Autodesk Inventor part; units mm, degrees
ref_plane "YZ Plane" through (0, 0, 0) normal (1, 0, 0) x (0, 1, 0)
ref_plane "XZ Plane" through (0, 0, 0) normal (0, 1, 0) x (-1, 0, 0)
ref_plane "XY Plane" through (0, 0, 0) normal (0, 0, 1) x (1, 0, 0)
sketch "スケッチ1" plane through (0, 0, 0) normal (0, 0, 1) x (1, 0, 0)
  line L0 (-12.25, 11.25) -> (12.25, 11.25)
  line L1 (14.25, 9.25) -> (14.25, -33.25)
  line L2 (12.25, -35.25) -> (-12.25, -35.25)
  line L3 (-14.25, -33.25) -> (-14.25, 9.25)
  line L4 (-12.25, 11.25) -> (-14.25, 9.25)
  line L5 (12.25, 11.25) -> (14.25, 9.25)
  line L6 (14.25, -33.25) -> (12.25, -35.25)
  line L7 (-12.25, -35.25) -> (-14.25, -33.25)
  line L8 (0, 0) -> (-26.5626, 0) construction
  line L9 (0, 0) -> (0, 27.9433) construction
  line L10 (-11, 8) -> (11, 8) construction
  line L11 (11, 8) -> (11, -32) construction
  line L12 (11, -32) -> (-11, -32) construction
  line L13 (-11, -32) -> (-11, 8) construction
  line L14 (-13.15, -28.5) -> (-13.15, 4.5)
  line L15 (-7.5, 10.15) -> (7.5, 10.15)
  line L16 (13.15, 4.5) -> (13.15, -28.5)
  line L17 (7.5, -34.15) -> (-7.5, -34.15)
  line L18 (8.5, 8) -> (8.5, 9.15)
  line L19 (11, 5.5) -> (12.15, 5.5)
  arc A0 (8.5, 8) -> (11, 5.5) centre (11, 8) ccw
  line L20 (12.15, -29.5) -> (11, -29.5)
  line L21 (8.5, -32) -> (8.5, -33.15)
  arc A1 (11, -29.5) -> (8.5, -32) centre (11, -32) ccw
  line L22 (-8.5, 8) -> (-8.5, 9.15)
  line L23 (-11, 5.5) -> (-12.15, 5.5)
  arc A2 (-11, 5.5) -> (-8.5, 8) centre (-11, 8) ccw
  line L24 (-12.15, -29.5) -> (-11, -29.5)
  line L25 (-8.5, -32) -> (-8.5, -33.15)
  arc A3 (-8.5, -32) -> (-11, -29.5) centre (-11, -32) ccw
  arc A4 (8.5, 9.15) -> (7.5, 10.15) centre (7.5, 9.15) ccw
  arc A5 (13.15, 4.5) -> (12.15, 5.5) centre (12.15, 4.5) ccw
  arc A6 (12.15, -29.5) -> (13.15, -28.5) centre (12.15, -28.5) ccw
  arc A7 (7.5, -34.15) -> (8.5, -33.15) centre (7.5, -33.15) ccw
  arc A8 (-8.5, -33.15) -> (-7.5, -34.15) centre (-7.5, -33.15) ccw
  arc A9 (-13.15, -28.5) -> (-12.15, -29.5) centre (-12.15, -28.5) ccw
  arc A10 (-12.15, 5.5) -> (-13.15, 4.5) centre (-12.15, 4.5) ccw
  arc A11 (-7.5, 10.15) -> (-8.5, 9.15) centre (-7.5, 9.15) ccw
  point P0 (-14.25, 11.25)
  point P1 (14.25, -35.25)
  point P2 (14.25, 11.25)
  point P3 (-14.25, -35.25)
  point P4 (8.5, 10.15)
  point P5 (13.15, 5.5)
  point P6 (13.15, -29.5)
  point P7 (8.5, -34.15)
  point P8 (-8.5, 10.15)
  point P9 (-13.15, 5.5)
  point P10 (-13.15, -29.5)
  point P11 (-8.5, -34.15)
  dimension "d0" = 2
  dimension "d1" = 2
  dimension "d2" = 2
  dimension "d3" = 2
  dimension "d4" = 2
  dimension "d5" = 2
  dimension "d6" = 2
  dimension "d7" = 2
  dimension "d8" = 28.5
  dimension "d9" = 11.25
  dimension "d10" = 46.5
  dimension "d11" = 8
  dimension "d12" = 22
  dimension "d13" = 40
  dimension "d14" = 1.1
  dimension "d15" = 2.5
  dimension "d16" = 2.5
  dimension "d17" = 1.1
  dimension "d18" = 1.1
  dimension "d19" = 1
extrude "押し出し1" add sketch "スケッチ1" along normal blind 3.1
hole "穴1" at (-11, 8, 0) at (11, 8, 0) at (11, -32, 0) at (-11, -32, 0) direction (0, 0, 1) diameter 2.5 end through all
sketch "スケッチ3" plane through (0, 0, 0) normal (0, 0, -1) x (-1, 0, 0)
  line L0 (-12.25, 11.25) -> (12.25, 11.25) construction
  line L1 (12.25, 11.25) -> (14.25, 9.25) construction
  line L2 (14.25, 9.25) -> (14.25, -33.25) construction
  line L3 (14.25, -33.25) -> (12.25, -35.25) construction
  line L4 (12.25, -35.25) -> (-12.25, -35.25) construction
  line L5 (-12.25, -35.25) -> (-14.25, -33.25) construction
  line L6 (-14.25, -33.25) -> (-14.25, 9.25) construction
  line L7 (-14.25, 9.25) -> (-12.25, 11.25) construction
  line L8 (11.087, 10.625) -> (-11.087, 10.625)
  line L9 (-11.9911, 10.625) -> (-13.625, 8.9911) construction
  line L10 (-13.625, 8.087) -> (-13.625, -32.087)
  line L11 (-13.625, -32.9911) -> (-11.9911, -34.625) construction
  line L12 (-11.087, -34.625) -> (11.087, -34.625)
  line L13 (11.9911, -34.625) -> (13.625, -32.9911) construction
  line L14 (13.625, -32.087) -> (13.625, 8.087)
  line L15 (13.625, 8.9911) -> (11.9911, 10.625) construction
  line L16 (-13.1857, -33.1476) -> (-12.1476, -34.1857)
  line L17 (12.1476, -34.1857) -> (13.1857, -33.1476)
  line L18 (12.1476, 10.1857) -> (13.1857, 9.1476)
  line L19 (-13.1857, 9.1476) -> (-12.1476, 10.1857)
  arc A0 (-13.1857, 9.1476) -> (-13.625, 8.087) centre (-12.125, 8.087) ccw
  arc A1 (-11.087, 10.625) -> (-12.1476, 10.1857) centre (-11.087, 9.125) ccw
  arc A2 (12.1476, 10.1857) -> (11.087, 10.625) centre (11.087, 9.125) ccw
  arc A3 (13.625, 8.087) -> (13.1857, 9.1476) centre (12.125, 8.087) ccw
  arc A4 (13.1857, -33.1476) -> (13.625, -32.087) centre (12.125, -32.087) ccw
  arc A5 (11.087, -34.625) -> (12.1476, -34.1857) centre (11.087, -33.125) ccw
  arc A6 (-12.1476, -34.1857) -> (-11.087, -34.625) centre (-11.087, -33.125) ccw
  arc A7 (-13.625, -32.087) -> (-13.1857, -33.1476) centre (-12.125, -32.087) ccw
  arc A8 (-12.15, 5.5) -> (-13.15, 4.5) centre (-12.15, 4.5) ccw
  line L20 (-12.15, 5.5) -> (-11, 5.5)
  arc A9 (-11, 5.5) -> (-8.5, 8) centre (-11, 8) ccw
  line L21 (-8.5, 8) -> (-8.5, 9.15)
  arc A10 (-7.5, 10.15) -> (-8.5, 9.15) centre (-7.5, 9.15) ccw
  line L22 (-7.5, 10.15) -> (7.5, 10.15)
  arc A11 (8.5, 9.15) -> (7.5, 10.15) centre (7.5, 9.15) ccw
  line L23 (8.5, 9.15) -> (8.5, 8)
  arc A12 (8.5, 8) -> (11, 5.5) centre (11, 8) ccw
  line L24 (11, 5.5) -> (12.15, 5.5)
  arc A13 (13.15, 4.5) -> (12.15, 5.5) centre (12.15, 4.5) ccw
  circle A14 centre (11, 8) radius 1.25
  line L25 (13.15, 4.5) -> (13.15, -28.5)
  arc A15 (12.15, -29.5) -> (13.15, -28.5) centre (12.15, -28.5) ccw
  line L26 (12.15, -29.5) -> (11, -29.5)
  arc A16 (11, -29.5) -> (8.5, -32) centre (11, -32) ccw
  line L27 (8.5, -32) -> (8.5, -33.15)
  arc A17 (7.5, -34.15) -> (8.5, -33.15) centre (7.5, -33.15) ccw
  circle A18 centre (11, -32) radius 1.25
  line L28 (7.5, -34.15) -> (-7.5, -34.15)
  arc A19 (-8.5, -33.15) -> (-7.5, -34.15) centre (-7.5, -33.15) ccw
  line L29 (-8.5, -33.15) -> (-8.5, -32)
  arc A20 (-8.5, -32) -> (-11, -29.5) centre (-11, -32) ccw
  line L30 (-11, -29.5) -> (-12.15, -29.5)
  arc A21 (-13.15, -28.5) -> (-12.15, -29.5) centre (-12.15, -28.5) ccw
  circle A22 centre (-11, -32) radius 1.25
  line L31 (-13.15, -28.5) -> (-13.15, 4.5)
  circle A23 centre (-11, 8) radius 1.25
  point P0 (0, 0)
  dimension "d30" = 0.625
  dimension "d31" = 1.5
  dimension "d32" = 0.2
extrude "押し出し2" add sketch "スケッチ3" along normal blind 0.75
properties part number "COXA_YAW_ROLL_ADPT_SPACER_2"
Work out the finished part from the listing and answer in its coordinate system (mm). A direction names the side the tool comes from. Coordinates: 2 decimals unless noted, no trailing zeros. Write each loop counter-clockwise with the first axis right and the second up, starting at its lowest first coordinate (ties: lowest second). Pieces come first, ordered by that corner, then holes. Notation, with made-up numbers: M 79.5,10.25 L 120.5,10.25 A22 ccw 120.5,19.25 Z; hole C 42,-25.5 d7. An arc over 180 degrees is marked long. Use one line per item in the form item = value. Start each with the question number.
1. Straight lines are drawn through the part: probe 1 along X at (y, z) = (8, 0.65); probe 2 along Y at (x, z) = (-11, 0.95); probe 3 along X at (y, z) = (8, -0.3) (3 decimals). For each, find the intervals that lie inside material, in ascending order. Write a range as from..to.
2. This flat-tipped pin is pushed along its axis until it touches: P1, Ø0.8, axis at x = 2.5, z = -0.5, coming from the -Y side (3 decimals). Where does it stop, or does it pass through?
3. The mould has two halves that part along Y. Classify faces 1 (the face through (12, 5.5, 1)), 2 (the face through (13.2, 10.3, 1.5)), 3 (the face through (9.9, -31.41, 1.2)), 4 (the face through (-14.25, -12, 2)): released by +Y, released by -Y, zero draft, split by the parting line, or undercut.
4. The part is cut by section C-C (z = 1.5). Give the number of separate pieces and of enclosed holes in the cut face, plus the area to 3 significant figures.
5. The part is cut by section A-A (y = -16.5). Give the vertices of the cut face in (x, z) (3 decimals).
6. A tool of negligible diameter and unlimited length cuts with its end or side. For faces 5 (the face through (12.674, -33.659, -0.37)), 6 (the face through (-12, -29.5, 1)), 7 (the face through (-12.659, -33.674, -0.37)), 8 (the face through (12.674, 9.659, -0.37)), 9 (the face through (-12.659, 9.674, -0.37)), from which of +Z, -Z, +X, -X, +Y, -Y can it reach the whole face along a straight path? Write none if from no direction.
7. The part is cut by section B-B (x = -2.5). Give the vertices of the cut face in (y, z) (3 decimals), plus the area to 3 significant figures.
Evaluation:
q1.probe_1 = -14.25..-12.25, -9.75..-8.5, 8.5..9.75, 12.25..14.25
q1.probe_2 = -35.25..-33.25, -30.75..-29.5, 5.5..6.75, 9.25..11.25
q1.probe_3 = -13.625..-12.25, -9.75..-8.5, 8.5..9.75, 12.25..13.625
q2.P1 = -34.625
q3.face_1 = undercut
q3.face_2 = released by +Y
q3.face_3 = undercut
q3.face_4 = zero draft
q4.separate_pieces = 1
q4.enclosed_holes = 5
q4.area = 215 mm^2
q5.outline = M -14.25,0 L -13.625,0 L -13.625,-0.75 L -13.15,-0.75 L -13.15,3.1 L -14.25,3.1 Z; M 13.15,-0.75 L 13.625,-0.75 L 13.625,0 L 14.25,0 L 14.25,3.1 L 13.15,3.1 Z
q6.face_5 = -Z, +X, -Y
q6.face_6 = +Z, -Z
q6.face_7 = -Z, -X, -Y
q6.face_8 = -Z, +X, +Y
q6.face_9 = -Z, -X, +Y
q7.outline = M -35.25,0 L -34.625,0 L -34.625,-0.75 L -34.15,-0.75 L -34.15,3.1 L -35.25,3.1 Z; M 10.15,-0.75 L 10.625,-0.75 L 10.625,0 L 11.25,0 L 11.25,3.1 L 10.15,3.1 Z
q7.area = 7.53 mm^2
